Drawing for the job (mm, zero at the part's lowest x, y, z). A direction names the side the tool comes from. Give positions to 0.01 mm unless a question says otherwise; leave off trailing zeros. Write each loop counter-clockwise with the first axis right and the second up, starting at its lowest first coordinate (ties: lowest second). Pieces come first, ordered by that corner, then holes. Notation, with made-up numbers: M 53,29.5 L 94,29.5 A25 ccw 94,67.5 Z; hole C 49.5,2.5 d6. An arc over 180 degrees is marked long. Write item = value, one per line. Start each with the question number.
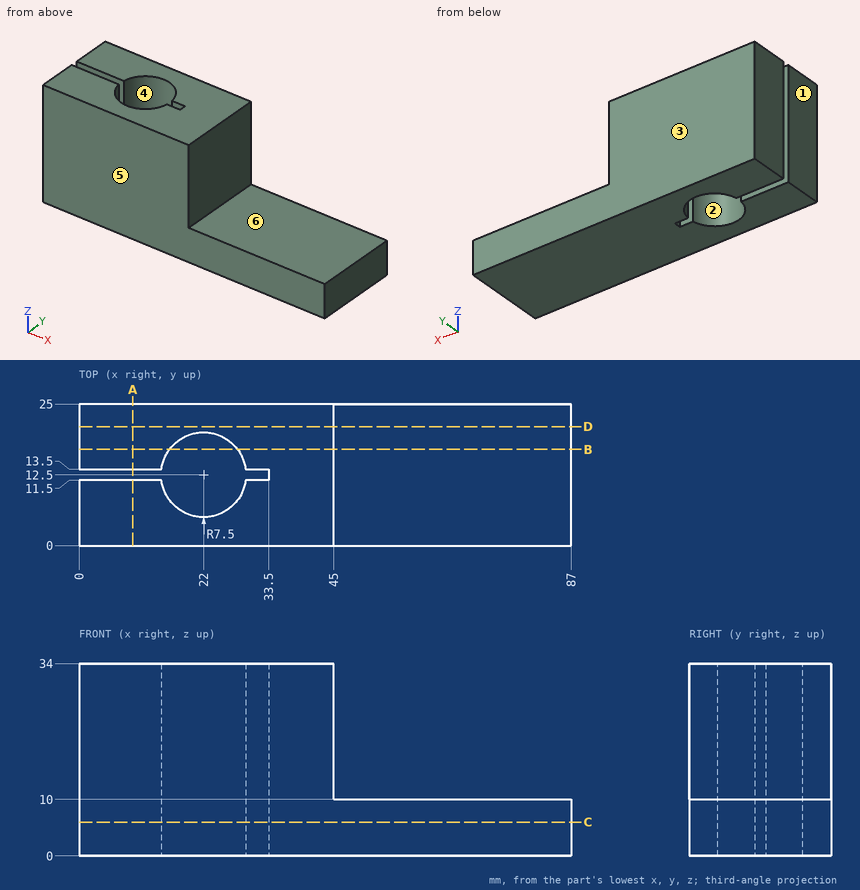
Q1. Drop flat-ended pins along their axis: P1, Ø4, axis at y = 16, z = 23.5, coming from the +X side; P2, Ø2, axis at x = 76.5, y = 9, coming from the +Z side; P3, Ø3, axis at x = 24.5, y = 8, coming from the +Z side. Give the stop position or say it passes through.
Q2. Slice it at A-A (x = 9.5). Give the cut face in (y, z).
Q3. Two-plate mould, pull along X, no slides. Class the marked faces 1, 2 and 3: +X half, -X half, draft (parallel to the pull), parting line (faces both ways), or undercut.
Q4. Slice it at D-D (y = 21). Give the cut face in (x, z), and give its area (3 significant figures).
Q5. Probe line 1 along X through (y, z) = (20.5, 28); line 2 along Z through (x, y) = (69, 8.25); line 3 along Y through (x, z) = (11.5, 12). List the from-to ranges inside material, lowest first.
Q6. Tool access for the marked faces 4, 5 and 6: list every direction of +Z, -Z, +X, -X, +Y, -Y with a clear straight run to the whole face (end or side of a thin tool).
Q7. Slice it at C-C (z = 6). Give the cut face in (x, y).
Q8. Slice it at B-B (y = 17). Give the cut face in (x, z).
Working result:
q1.P1 = 45
q1.P2 = 10
q1.P3 = through
q2.outline = M 0,0 L 11.5,0 L 11.5,34 L 0,34 Z; M 13.5,0 L 25,0 L 25,34 L 13.5,34 Z
q3.face_1 = -X half
q3.face_2 = undercut
q3.face_3 = draft
q4.outline = M 0,0 L 87,0 L 87,10 L 45,10 L 45,34 L 0,34 Z
q4.area = 1,950 mm2
q5.line_1 = 0 to 45
q5.line_2 = 0 to 10
q5.line_3 = 0 to 11.5, 13.5 to 25
q6.face_4 = +Z, -Z
q6.face_5 = +Z, -Z, +X, -X, -Y
q6.face_6 = +Z, +X, +Y, -Y
q7.outline = M 0,0 L 87,0 L 87,25 L 0,25 L 0,13.5 L 14.57,13.5 A7.5 cw 29.43,13.5 L 33.5,13.5 L 33.5,11.5 L 29.43,11.5 A7.5 cw 14.57,11.5 L 0,11.5 Z
q8.outline = M 0,0 L 16,0 L 16,34 L 0,34 Z; M 28,0 L 87,0 L 87,10 L 45,10 L 45,34 L 28,34 Z
